Input: part model. Units: mm. Frame: model coordinates. Face numbers are marked on the shaded views. A direction names the side the tool comes from. Give positions to 0.01 mm unless a question says otherwise; leave off trailing zeros. Loops run counter-clockwise (first coordinate to the right, second up) from the corner with the lowest first, then second, coordinate; pieces in that order, holes last. Notation, with made-up numbers: (-22, 31.25) - (-17, 31.25) arc R9 ccw to (-17, 38.25) - close; hole circle Ø7 at (87.5, 13.5). An arc over 180 degrees is marked (long way). Answer as a JSON object with one key per item and string values. Group by question number.
(1) Section query A-A (x = -0.25). Return loops of the section in (y, z), plus the area to 3 significant figures.
(2) Mould query, pull axis Y, two halves, no side actions, for the marked faces 1, 2 and 3. Classes: +Y half, -Y half, draft (parallel to the pull), parting line (faces both ways), or undercut.
(3) Pin query (flat end, axial travel): P1, Ø6, axis at y = -5, z = 8.5, coming from the +X side. Return the tip coordinate at first contact, or that it passes through.
(4) Section query C-C (x = 2). Return loops of the section in (y, z).
(5) Section query B-B (z = 6). Return loops of the section in (x, y), plus the area to 3 significant figures.
(6) Material intervals for L1, parallel to Y at x = 1.75, z = 8.5; L2, parallel to X at y = 4, z = 10; L3, parallel to Y at x = 5.75, z = 10, sorted ascending.
(7) Section query D-D (z = 4.5). Return loops of the section in (x, y), plus the area to 3 significant figures.
(8) Access query for the marked faces 4 and 5. Directions: +Z, -Z, +X, -X, +Y, -Y. A direction counts if a zero-diameter tool reaches every point of the face in a straight line with its end or side. Return the directions, or none.
```python
from build123d import *
from OCP.BRepFilletAPI import BRepFilletAPI_MakeChamfer

# Parameters (mm, degrees)
SALIENTE_EXTRUIR1_DEPTH = 12
CROQUIS2_R              = 1.9
CORTAR_EXTRUIR1_DEPTH   = 35.077118423
REDONDEO1_R             = 0.5
REDONDEO2_R             = 2.5
CHAFL_N1_SIZE           = 1
CHAFL_N1_SIZE2          = 2.747477419


with BuildPart() as part:
    # Croquis1 → Saliente-Extruir1 (new body)
    with BuildSketch(Plane.XY):
        Polygon((-3.5, 11.5), (3.5, 11.5), (7.5, 11.5), (7.5, 15.5), (-7.5, 15.5), (-7.5, -15.5), (7.5, -15.5), (7.5, -11.5), (3.5, -11.5), (-3.5, -11.5), align=None)
    extrude(amount=SALIENTE_EXTRUIR1_DEPTH)

    # Croquis2 → Cortar-Extruir1 (cut, through all)
    with BuildSketch(Plane(origin=(0, 15.5, 0), x_dir=(1, 0, 0), z_dir=(0, 1, 0))):
        with Locations(Location((2, -6, 0), (0, 0, 270))):
            Circle(CROQUIS2_R)
    extrude(amount=-CORTAR_EXTRUIR1_DEPTH, mode=Mode.SUBTRACT)

    # Redondeo1
    redondeo1_edges = [part.edges().sort_by_distance(p)[0] for p in [
        (-3.5, 11.5, 6),
        (-3.5, -11.5, 6),
    ]]
    fillet(redondeo1_edges, radius=REDONDEO1_R)

    # Redondeo2
    redondeo2_edges = [part.edges().sort_by_distance(p)[0] for p in [
        (-7.5, -15.5, 6),
        (-7.5, 15.5, 6),
    ]]
    fillet(redondeo2_edges, radius=REDONDEO2_R)

    # Chaflán1: one chamfer whose edges measure the first distance from different faces: ONE call of the kernel's chamfer builder (chamfer() names one face for all edges)
    chafl_n1_edges_1 = [part.edges().sort_by_distance(p)[0] for p in [
        (7.5, -11.5, 6),
    ]]
    chafl_n1_side_1 = [part.faces().sort_by_distance(p)[0] for p in [
        (7.5, -13.5, 6),
    ]]
    chafl_n1_edges_2 = [part.edges().sort_by_distance(p)[0] for p in [
        (7.5, 11.5, 6),
    ]]
    chafl_n1_side_2 = [part.faces().sort_by_distance(p)[0] for p in [
        (7.5, 13.5, 6),
    ]]
    chafl_n1 = BRepFilletAPI_MakeChamfer(part.part.solid().wrapped)
    for e in chafl_n1_edges_1:
        chafl_n1.Add(CHAFL_N1_SIZE, CHAFL_N1_SIZE2, e.wrapped, chafl_n1_side_1[0].wrapped)  # the first distance lies on this face
    for e in chafl_n1_edges_2:
        chafl_n1.Add(CHAFL_N1_SIZE, CHAFL_N1_SIZE2, e.wrapped, chafl_n1_side_2[0].wrapped)  # the first distance lies on this face
    add(Compound.cast(chafl_n1.Shape()), mode=Mode.REPLACE)


solid = part.part
```
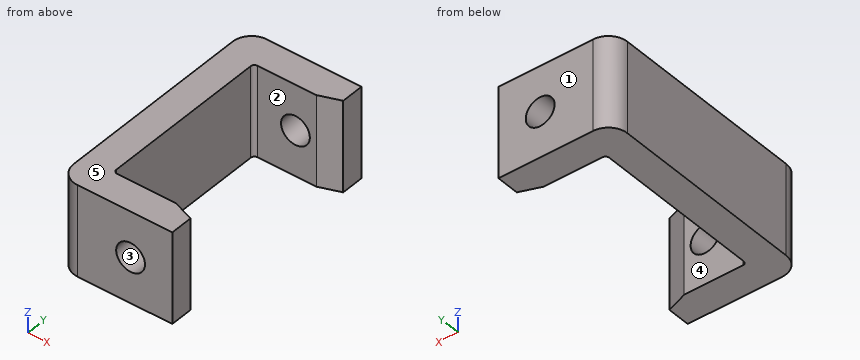
Recorded:
{
 "1": {"outline": "(-15.5, 0) - (-11.5, 0) - (-11.5, 12) - (-15.5, 12) - close; (11.5, 0) - (15.5, 0) - (15.5, 12) - (11.5, 12) - close", "area": "96.0 mm^2"},
 "2": {"face 1": "+Y half", "face 2": "undercut", "face 3": "draft"},
 "3": {"P1": "stops at x = -3.5"},
 "4": {"outline": "(-15.5, 0) - (-11.5, 0) - (-11.5, 4.1) - (-15.5, 4.1) - close; (-15.5, 7.9) - (-11.5, 7.9) - (-11.5, 12) - (-15.5, 12) - close; (11.5, 0) - (15.5, 0) - (15.5, 4.1) - (11.5, 4.1) - close; (11.5, 7.9) - (15.5, 7.9) - (15.5, 12) - (11.5, 12) - close"},
 "5": {"outline": "(-7.5, -13) arc R2.5 ccw to (-5, -15.5) - (0.1, -15.5) - (0.1, -11.5) - (-3, -11.5) arc R0.5 cw to (-3.5, -11) - (-3.5, 11) arc R0.5 cw to (-3, 11.5) - (0.1, 11.5) - (0.1, 15.5) - (-5, 15.5) arc R2.5 ccw to (-7.5, 13) - close; (3.9, -15.5) - (7.5, -15.5) - (7.5, -12.5) - (4.75, -11.5) - (3.9, -11.5) - close; (3.9, 11.5) - (4.75, 11.5) - (7.5, 12.5) - (7.5, 15.5) - (3.9, 15.5) - close", "area": "176 mm^2"},
 "6": {"L1": "y = -15.5 to -11.5, 11.5 to 15.5", "L2": "x = -7.5 to -3.5", "L3": "y = -15.5 to -11.86, 11.86 to 15.5"},
 "7": {"outline": "(-7.5, -13) arc R2.5 ccw to (-5, -15.5) - (0.83, -15.5) - (0.83, -11.5) - (-3, -11.5) arc R0.5 cw to (-3.5, -11) - (-3.5, 11) arc R0.5 cw to (-3, 11.5) - (0.83, 11.5) - (0.83, 15.5) - (-5, 15.5) arc R2.5 ccw to (-7.5, 13) - close; (3.17, -15.5) - (7.5, -15.5) - (7.5, -12.5) - (4.75, -11.5) - (3.17, -11.5) - close; (3.17, 11.5) - (4.75, 11.5) - (7.5, 12.5) - (7.5, 15.5) - (3.17, 15.5) - close", "area": "188 mm^2"},
 "8": {"face 4": "+Z, -Z, +X", "face 5": "+Z, +X, -X, +Y, -Y"}
}
